from build123d import *

# Parameters (mm, degrees)
SKETCH1_W           = 70
SKETCH1_H           = 40
SKETCH1_R           = 3
BOSS_EXTRUDE1_DEPTH = 3.1
SKETCH2_W           = 3.1
SKETCH2_H           = 20
BOSS_EXTRUDE2_DEPTH = 3.1


with BuildPart() as part:
    # Sketch1 → Boss-Extrude1 (new body)
    with BuildSketch(Plane.XY):
        Rectangle(SKETCH1_W, SKETCH1_H)
        with Locations((-6, 0)):
            Circle(SKETCH1_R, mode=Mode.SUBTRACT)
        with Locations((0, 6)):
            Circle(SKETCH1_R, mode=Mode.SUBTRACT)
        with Locations((6, 0)):
            Circle(SKETCH1_R, mode=Mode.SUBTRACT)
        with Locations((0, -6)):
            Circle(SKETCH1_R, mode=Mode.SUBTRACT)
    extrude(amount=BOSS_EXTRUDE1_DEPTH)

    # Sketch2 → Boss-Extrude2 (add, through all)
    with BuildSketch(Plane.XY.offset(3.1)):
        with Locations((36.55, -10)):
            Rectangle(SKETCH2_W, SKETCH2_H)
        with Locations((-36.55, -10)):
            Rectangle(SKETCH2_W, SKETCH2_H)
    extrude(amount=-BOSS_EXTRUDE2_DEPTH)


solid = part.part
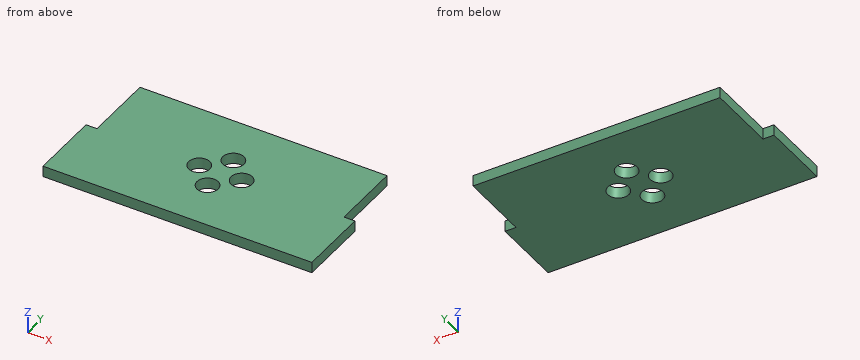
Design review of the part built by this model. Coordinates are the model's own, in mm. Round coordinates to 2 decimals unless told otherwise and drop trailing zeros. Loops run counter-clockwise (first coordinate to the right, second up) from the corner with the lowest first, then second, coordinate; pieces in that order, holes last. Notation, with made-up numbers: (87, -8) - (117, -8) arc R21 ccw to (117, -1) - close; hole circle Ø4 at (48.25, 19.25). An arc over 180 degrees is marked (long way). One line per item, written item: value. Start each with the question number.
1) Insertion check: pin 1 Ø1 at (y, z) = (10.5, 2) entering from -X; pin 2 Ø1.5 at (x, z) = (37, 1.5) entering from +Y. Each pin has a flat end and moves straight along its axis. Give the tip position at first contact, or say it passes through.
2) Consider section C-C on z = 0.5. Give the boundary of the cut face in (x, y).
3) To check wall thickness, follow L1, parallel to Y at x = 0, z = 1.9; L2, parallel to X at y = 1, z = 2.95; L3, parallel to Y at x = 6, z = 2.25. State the ranges of each line that lie inside material, in increasing order. Write a range as from..to.
4) Consider section B-B on x = 0. Give the boundary of the cut face in (y, z).
5) Consider section A-A on y = -6. Give the boundary of the cut face in (x, z), then the cut area to 3 significant figures.
6) Consider section D-D on y = 6. Give the boundary of the cut face in (x, z), then the cut area to 3 significant figures.
Reported:
1. pin 1: stops at x = -35
1. pin 2: stops at y = 0
2. outline: (-38.1, -20) - (38.1, -20) - (38.1, 0) - (35, 0) - (35, 20) - (-35, 20) - (-35, 0) - (-38.1, 0) - close; hole circle Ø6 at (-6, 0); hole circle Ø6 at (0, -6); hole circle Ø6 at (0, 6); hole circle Ø6 at (6, 0)
3. L1: y = -20..-9, -3..3, 9..20
3. L2: x = -35..-8.83, -3.17..3.17, 8.83..35
3. L3: y = -20..-3, 3..20
4. outline: (-20, 0) - (-9, 0) - (-9, 3.1) - (-20, 3.1) - close; (-3, 0) - (3, 0) - (3, 3.1) - (-3, 3.1) - close; (9, 0) - (20, 0) - (20, 3.1) - (9, 3.1) - close
5. outline: (-38.1, 0) - (-3, 0) - (-3, 3.1) - (-38.1, 3.1) - close; (3, 0) - (38.1, 0) - (38.1, 3.1) - (3, 3.1) - close
5. area: 218 mm^2
6. outline: (-35, 0) - (-3, 0) - (-3, 3.1) - (-35, 3.1) - close; (3, 0) - (35, 0) - (35, 3.1) - (3, 3.1) - close
6. area: 198 mm^2
